from build123d import *

# Parameters (mm, degrees)
BLANK_BEFORE_THREAD_DEPTH      = 1.778
BLANK_BEFORE_THREAD_DEPTH_BACK = 5.334
SKETCH1_R                      = 11.1125
SKETCH4_R                      = 11.938
HEAD_DEPTH                     = 1.778
RECESS_START                   = -1.27
SKETCH5_R                      = 11.938
SKETCH5_R_2                    = 10.1346
RECESS_UNDER_HEAD_DEPTH        = 1.27
FILL_START                     = 1.27
SKETCH8_R                      = 10.1346
FILL_IN_RECESS_DEPTH           = 1.27
HEX_THRU_DEPTH                 = 19.319722487
FILLET_ON_HEX_R                = 1.27
SKETCH7_R                      = 8.128
SKETCH7_R_2                    = 5.3594
SPRING_RECESS_DEPTH            = 5.334
SPRING_RECESS_DRAFT            = -2
FILLET1_R                      = 0.508


with BuildPart() as part:
    # Sketch1 → Blank Before Thread (new, two sides: drawn at the far end of the back side and taken through both)
    with BuildSketch(Plane(origin=(0, 0, 0), x_dir=(1, 0, 0), z_dir=(0, 1, 0)).offset(-BLANK_BEFORE_THREAD_DEPTH_BACK)):
        with Locations(Location((0, 0, 0), (0, 0, 270))):
            Circle(SKETCH1_R)
    extrude(amount=BLANK_BEFORE_THREAD_DEPTH + BLANK_BEFORE_THREAD_DEPTH_BACK)

    # Sketch4 → Head (add)
    with BuildSketch(Plane(origin=(0, 0, 0), x_dir=(1, 0, 0), z_dir=(0, 1, 0))):
        with Locations(Location((0, 0, 0), (0, 0, 270))):
            Circle(SKETCH4_R)
    extrude(amount=HEAD_DEPTH)

    # Sketch5 → Recess Under Head (cut)
    with BuildSketch(Plane(origin=(0, 0, 0), x_dir=(1, 0, 0), z_dir=(0, 1, 0)).offset(RECESS_START)):
        with Locations(Location((0, 0, 0), (0, 0, 270))):
            Circle(SKETCH5_R)
        with Locations(Location((0, 0, 0), (0, 0, 270))):
            Circle(SKETCH5_R_2, mode=Mode.SUBTRACT)
    extrude(amount=RECESS_UNDER_HEAD_DEPTH, mode=Mode.SUBTRACT)

    # Sketch8 → Fill in Recess (add)
    with BuildSketch(Plane.XZ.offset(FILL_START)):
        with Locations(Location((0, 0, 0), (0, 0, 90))):
            Circle(SKETCH8_R)
    extrude(amount=-FILL_IN_RECESS_DEPTH)

    # Sketch6 → Hex Thru (cut, through all)
    with BuildSketch(Plane(origin=(0, 1.778, 0), x_dir=(-1, 0, 0), z_dir=(0, 1, 0))):
        Polygon((1.957737028, -3.3909), (-1.957737028, -3.3909), (-3.915474056, 0), (-1.957737028, 3.3909), (1.957737028, 3.3909), (3.915474056, 0), align=None)
    extrude(amount=-HEX_THRU_DEPTH, mode=Mode.SUBTRACT)

    # Fillet on Hex
    fillet_on_hex_edges = [part.edges().sort_by_distance(p)[0] for p in [
        (2.936605542, 1.778, -1.69545),
        (-2.936605542, 1.778, 1.69545),
        (0, 1.778, -3.3909),
        (-2.936605542, 1.778, -1.69545),
        (0, 1.778, 3.3909),
        (2.936605542, 1.778, 1.69545),
    ]]
    fillet(fillet_on_hex_edges, radius=FILLET_ON_HEX_R)


with BuildPart() as spring_recess_tool:
    # Sketch7 → Spring Recess (with draft: the straight prism first)
    with BuildSketch(Plane(origin=(0, 1.778, 0), x_dir=(-1, 0, 0), z_dir=(0, 1, 0))):
        Circle(SKETCH7_R)
        Circle(SKETCH7_R_2, mode=Mode.SUBTRACT)
    extrude(amount=-SPRING_RECESS_DEPTH)
    # Spring Recess: the draft: its side faces are tilted about the plane it starts from
    spring_recess_sides = [spring_recess_tool.faces().sort_by_distance(p)[0] for p in [
        (8.128, -0.889, 0),
        (5.3594, -0.889, 0),
    ]]
    draft(spring_recess_sides, Plane(origin=(0, 1.778, 0), x_dir=(-1, 0, 0), z_dir=(0, 1, 0)), SPRING_RECESS_DRAFT)


with BuildPart() as part_1:
    add(part.part)

    # Spring Recess: cut by spring_recess_tool
    add(spring_recess_tool.part, mode=Mode.SUBTRACT)

    # Fillet1
    fillet1_edges = [part_1.edges().sort_by_distance(p)[0] for p in [
        (7.941732616, -3.556, 0),
        (5.545667384, -3.556, 0),
    ]]
    fillet(fillet1_edges, radius=FILLET1_R)


solid = part_1.part
Source: CAD feature listing. Evaluate the final solid. Frame: model axes, mm. A direction names the side the tool comes from. Round coordinates to 2 decimals unless told otherwise and drop trailing zeros. Loops run counter-clockwise (first coordinate to the right, second up) from the corner with the lowest first, then second, coordinate; pieces in that order, holes last.
Q1. Mould query, pull axis X, two halves, no side actions, for faces 1 (the face through (0, -2, -3.391)), 2 (the face through (-2.95, -2.37, -1.67)), 3 (the face through (-4, 1.778, -3)), 4 (the face through (3.04, -0.64, 9.67)). Classes: pulls with the +X half, pulls with the -X half, needs draft (parallel to the pull), parting line crosses it, or undercut.
Q2. Access query for faces 5 (the face through (3, -5.334, 2)), 6 (the face through (-2.923, -2.372, 1.719)), 7 (the face through (-3.25, 1.42, -1.92)), 8 (the face through (4, 1.778, -3)), 9 (the face through (-9, 0, -5)). Directions: +Z, -Z, +X, -X, +Y, -Y. A direction counts if a zero-diameter tool reaches every point of the face in a straight line with its end or side. Return the directions, or none.
Q3. First-contact query: P1, Ø4, axis at y = -2, z = -9.5, coming from the +X side; P2, Ø2, axis at x = -1, y = -3.5, coming from the -Z side; P3, Ø1.5, axis at x = -1.5, y = -1, coming from the +Z side. Flat tips, straight axial feed; report the tip coordinate or a pass-through.
Q4. Section D-D, the plane x = 9.5. Return loops of the section in (y, z).
Q5. Section B-B, the plane y = -2.5. Return loops of the section in (x, z) (1 decimal), plus the area to 3 significant figures.
Q6. Section C-C, the plane x = -9.75. Return loops of the section in (y, z).
Q7. Ray query, line 1 (Z direction, x = -2.75, y = -3.25); line 2 (X direction, y = 0.5, z = -4.25); line 3 (X direction, y = -2.75, z = -2.75). Return the intervals inside material, ascending.
Solutions:
1. face 1: undercut
1. face 2: undercut
1. face 3: needs draft
1. face 4: parting line crosses it
2. face 5: +Z, -Z, +X, -X, -Y
2. face 6: +Y, -Y
2. face 7: +Y
2. face 8: +Z, -Z, +X, -X, +Y
2. face 9: none
3. P1: stops at x = 8.2
3. P2: stops at z = -11.11
3. P3: stops at z = 11.08
4. outline: (-5.33, -5.77) - (-1.27, -5.77) - (-1.27, -3.53) - (0, -3.53) - (0, -7.23) - (1.78, -7.23) - (1.78, 7.23) - (0, 7.23) - (0, 3.53) - (-1.27, 3.53) - (-1.27, 5.77) - (-5.33, 5.77) - close
5. outline: circle Ø22.2 at (0, 0); circle Ø11 at (0, 0); hole circle Ø16 at (0, 0); hole (-3.9, 0) - (-2, -3.4) - (2, -3.4) - (3.9, 0) - (2, 3.4) - (-2, 3.4) - close
5. area: 243 mm2
6. outline: (-5.33, -5.33) - (-1.27, -5.33) - (-1.27, -2.77) - (0, -2.77) - (0, -6.89) - (1.78, -6.89) - (1.78, 6.89) - (0, 6.89) - (0, 2.77) - (-1.27, 2.77) - (-1.27, 5.33) - (-5.33, 5.33) - close
7. line 1: z = -10.77 to -7.42, -4.84 to -2.02, 2.02 to 4.84, 7.42 to 10.77
7. line 2: x = -11.16 to -6.88, -3.34 to 3.34, 6.88 to 11.16
7. line 3: x = -10.77 to -7.48, -4.78 to -2.33, 2.33 to 4.78, 7.48 to 10.77
